Answer from the drawing. Dimensions are ordinates in mm from the lowest x, y and z of the part. A direction names the side the tool comes from. Round coordinates to 2 decimals unless told otherwise and drop trailing zeros. Loops run counter-clockwise (first coordinate to the right, second up) from the corner with the lowest first, then second, coordinate; pieces in that order, holes last. Notation, with made-up numbers: (61.5, 27) - (77.5, 27) arc R9 ccw to (77.5, 44) - close; hole circle Ø4 at (46, 35). An arc over 180 degrees is marked (long way). Answer as CSV lines item,"result". Start each with the question number.
Q1. This flat-tipped pin is pushed along its axis until it touches: pin 1 Ø10 at (x, z) = (24, 69.5) entering from +Y. Where does it stop, or does it pass through?
Q2. Section D-D on y = 122 is taken. Write down the section's boundary in (x, z).
Q3. For the marked faces 5 and 6, determine the directions among +Z, -Z, +X, -X, +Y, -Y from which every point of the face is accessible in a straight line to the end or side of a thin tool.
Q4. The mould has two halves that part along Z. Classify the marked faces 1, 2, 3 and 4: +Z half, -Z half, draft (parallel to the pull), parting line (faces both ways), or undercut.
Q5. Section C-C on z = 60 is taken. Write down the section's boundary in (x, y).
Q6. Section A-A on y = 70 is taken. Write down the section's boundary in (x, z), then the cut area to 3 significant figures.
Q7. Section B-B on x = 12 is taken. Write down the section's boundary in (y, z), then the cut area to 3 significant figures.
Q8. Straight lines are drawn through the part: L1, parallel to Y at x = 19, z = 73.5; L2, parallel to Y at x = 8, z = 46.5; L3, parallel to Z at x = 17.5, y = 118.5. For each, find the intervals that lie inside material, in ascending order. Write a range as [from, to].
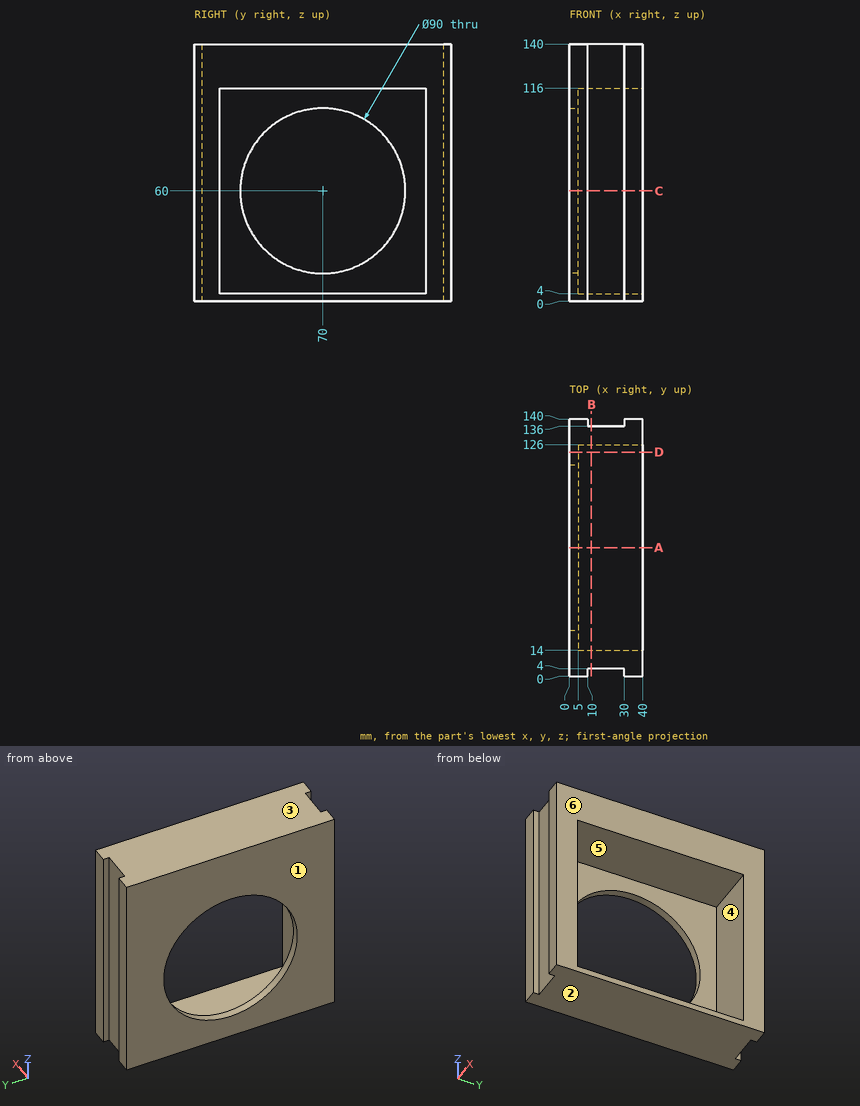
Findings:
1,pin 1,"stops at y = 136"
2,outline,"(0, 0) - (40, 0) - (40, 4) - (5, 4) - (5, 116) - (40, 116) - (40, 140) - (0, 140) - close"
3,face 5,"+X"
3,face 6,"+Z, -Z, +X, +Y, -Y"
4,face 1,"draft"
4,face 2,"-Z half"
4,face 3,"+Z half"
4,face 4,"undercut"
5,outline,"(0, 0) - (10, 0) - (10, 4) - (30, 4) - (30, 0) - (40, 0) - (40, 14) - (5, 14) - (5, 25) - (0, 25) - close; (0, 115) - (5, 115) - (5, 126) - (40, 126) - (40, 140) - (30, 140) - (30, 136) - (10, 136) - (10, 140) - (0, 140) - close"
6,outline,"(0, 0) - (40, 0) - (40, 4) - (5, 4) - (5, 15) - (0, 15) - close; (0, 105) - (5, 105) - (5, 116) - (40, 116) - (40, 140) - (0, 140) - close"
6,area,"1,230 mm^2"
7,outline,"(4, 0) - (136, 0) - (136, 140) - (4, 140) - close; hole (14, 4) - (126, 4) - (126, 116) - (14, 116) - close"
7,area,"5,940 mm^2"
8,L1,"y = [4, 14], [126, 136]"
8,L2,"y = [0, 14], [126, 140]"
8,L3,"z = [0, 4], [116, 140]"
